from build123d import *

# Parameters (mm, degrees)
F0_W      = 38.1
F0_H      = 38.1
F1_DEPTH  = 38.1
F6_DEPTH  = 38.1
F8_DEPTH  = 38.1
F9_W      = 25.4
F9_H      = 7.62
F10_DEPTH = 38.1


with BuildPart() as f1:
    # F0 (on Front) → F1 (new body)
    with BuildSketch(Plane.XZ):
        with Locations((19.05, 19.05)):
            Rectangle(F0_W, F0_H)
    extrude(amount=F1_DEPTH)

    # F5 (on offset) → F6 (cut)
    with BuildSketch(Plane.YZ.offset(38.1)):
        Polygon((-11.43, 15.875), (-6.35, 38.1), (-31.75, 38.1), (-26.67, 15.875), (-21.59, 28.575), (-16.51, 28.575), align=None)
        Polygon((-25.4, 0), (-12.7, 0), (-19.05, 15.875), align=None)
        Polygon((-6.35, 0), (0, 0), (0, 38.1), align=None)
        Polygon((-31.75, 0), (-38.1, 38.1), (-38.1, 0), align=None)
    extrude(amount=-F6_DEPTH, mode=Mode.SUBTRACT)

    # F7 (on offset) → F8 (cut)
    with BuildSketch(Plane.XZ.offset(38.1)):
        Polygon((0, 38.1), (0, 0), (6.35, 38.1), align=None)
        Polygon((25.4, 38.1), (12.7, 38.1), (19.05, 29.0341), align=None)
        Polygon((31.75, 38.1), (38.1, 0), (38.1, 38.1), align=None)
        Polygon((11.43, 22.225), (6.35, 0), (31.75, 0), (26.67, 22.225), (21.59, 9.525), (16.51, 9.525), align=None)
    extrude(amount=-F8_DEPTH, mode=Mode.SUBTRACT)

    # F9 (on offset) → F10 (cut)
    with BuildSketch(Plane.XY.offset(38.1)):
        with Locations((25.4, -11.43)):
            Rectangle(F9_W, F9_H)
        with Locations((12.7, -26.67)):
            Rectangle(F9_W, F9_H)
    extrude(amount=-F10_DEPTH, mode=Mode.SUBTRACT)


solid = f1.part
Here's how the part is built. I have some questions about the finished solid (model axes, mm). A direction names the side the tool comes from. Coordinates: 2 decimals unless noted, no trailing zeros. Loops run counter-clockwise (first coordinate to the right, second up) from the corner with the lowest first, then second, coordinate; pieces in that order, holes last.
1. Imagine slicing it at C-C, the plane z = 3.5. Please give me the cut outline in (x, y), and give its area (3 significant figures).
2. For P1, Ø20.5, axis at x = 9.5, z = 15.5, coming from the +Y side; P2, Ø3, axis at y = -17.5, z = 26, coming from the -X side; P3, Ø3, axis at x = 31, z = 21, coming from the +Y side, each with a flat end and sliding along its axis, tell me the tip position at first contact or that it passes through.
3. Imagine slicing it at A-A, the plane z = 23. Please give me the cut outline in (x, y), and give its area (3 significant figures).
4. For faces 1 (the flat face through (19, -6, 9.525)), 2 (the flat face through (9.845, -31.124, 35.361)), 3 (the flat face through (12.7, -8, 23)), 4 (the flat face through (19.1, -20, 13.5)), 5 (the flat face through (15.83, -34.34, 33.63)), which set-ups out of +Z, -Z, +X, -X, +Y, -Y let a thin tool reach every point of the face, with its end or its side?
5. Imagine slicing it at B-B, the plane x = 12. Please give me the cut outline in (y, z) (3 decimals).
6. I need wall thicknesses on L1, parallel to Y at x = 33, z = 12; L2, parallel to Y at x = 34, z = 14; L3, parallel to X at y = -4, z = 15. Which ranges of each line are inside material? Lowest first, please.
7. Imagine slicing it at D-D, the plane y = -34.5. Please give me the cut outline in (x, z) (3 decimals).
8. If we mould it in two halves opening along Y, with no side actions, what happens to faces 6 (the flat face through (35, -29, 0)), 7 (the flat face through (13, -30.48, 20)), 8 (the flat face through (25.4, -24, 21))? For each: pulls with the +Y half, pulls with the -Y half, needs draft (parallel to the pull), parting line crosses it, or undercut.
Taken from the geometry:
1. outline: (0.58, -32.33) - (7.15, -32.33) - (7.15, -30.48) - (0.58, -30.48) - close; (0.58, -14.1) - (7.15, -14.1) - (7.15, -5.77) - (0.58, -5.77) - close; (30.95, -32.33) - (37.52, -32.33) - (37.52, -24) - (30.95, -24) - close; (30.95, -7.62) - (37.52, -7.62) - (37.52, -5.77) - (30.95, -5.77) - close
1. area: 134 mm2
2. P1: stops at y = -2.06
2. P2: stops at x = 4.08
2. P3: stops at y = -2.6
3. outline: (3.83, -35.58) - (34.27, -35.58) - (34.27, -28.3) - (25.4, -28.3) - (25.4, -30.48) - (3.83, -30.48) - close; (3.83, -22.86) - (25.4, -22.86) - (25.4, -23.82) - (34.27, -23.82) - (34.27, -15.24) - (12.7, -15.24) - (12.7, -14.28) - (3.83, -14.28) - close; (3.83, -9.8) - (12.7, -9.8) - (12.7, -7.62) - (34.27, -7.62) - (34.27, -2.52) - (3.83, -2.52) - close
3. area: 598 mm2
4. face 1: -Z, +Y, -Y
4. face 2: +Z, +X, -X
4. face 3: +Z, -Z, +X
4. face 4: -Z, +X, -X
4. face 5: +Z, +Y, -Y
5. outline: (-38.1, 38.1) - (-35.217, 20.8) - (-30.48, 20.8) - (-30.48, 32.544) - (-31.75, 38.1) - close; (-22.86, 20.8) - (-13.4, 20.8) - (-16.51, 28.575) - (-21.59, 28.575) - (-22.86, 25.4) - close; (-10.304, 20.8) - (-2.883, 20.8) - (0, 38.1) - (-6.35, 38.1) - close
6. L1: y = -33.75 to -20.6, -17.5 to -15.24, -7.62 to -4.35
6. L2: y = -34.08 to -19.8, -18.3 to -15.24, -7.62 to -4.02
6. L3: x = 2.5 to 9.78, 14.32 to 23.78, 28.32 to 35.6
7. outline: (2.75, 16.5) - (10.121, 16.5) - (11.43, 22.225) - (13.72, 16.5) - (24.38, 16.5) - (26.67, 22.225) - (27.979, 16.5) - (35.35, 16.5) - (31.75, 38.1) - (25.4, 38.1) - (19.05, 29.034) - (12.7, 38.1) - (6.35, 38.1) - close
8. face 6: needs draft
8. face 7: undercut
8. face 8: undercut
